Here's the drawing with two shaded views (mm, measured from the low corner). I have some questions. A direction names the side the tool comes from. Coordinates: 2 decimals unless noted, no trailing zeros. Write each loop counter-clockwise with the first axis right and the second up, starting at its lowest first coordinate (ties: lowest second). Pieces come first, ordered by that corner, then holes.
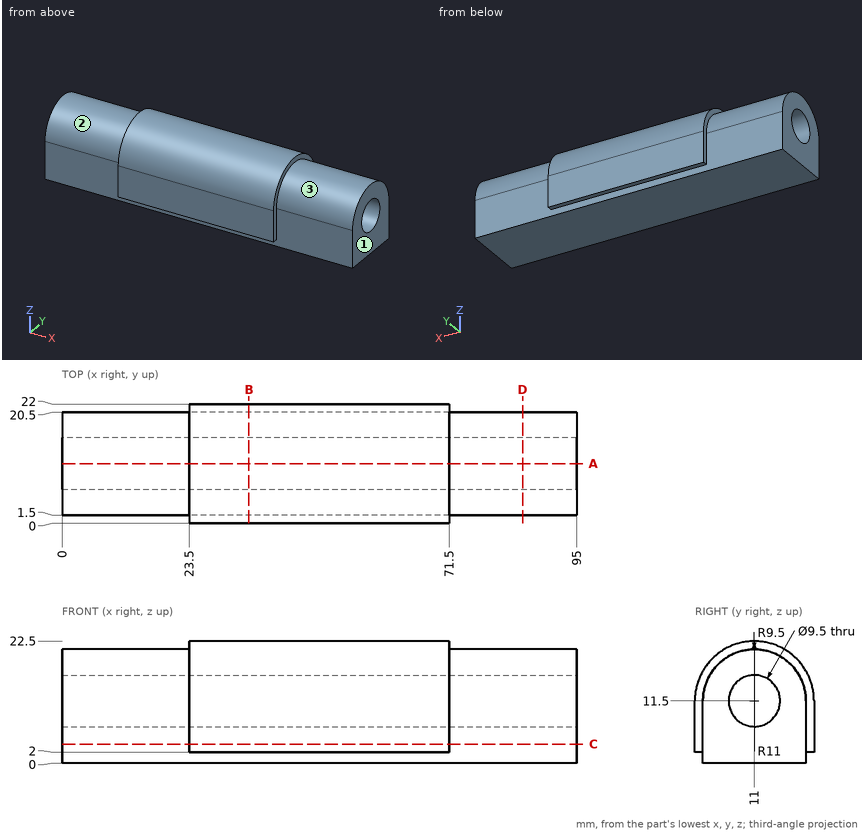
1. Which directions (+Z, -Z, +X, -X, +Y, -Y) give clear straight access to the entire face, cutting with the end or side of a thin tool? Please do the marked faces 1, 2 and 3.
2. If we section it at C-C, the plane z = 3.5: List the corners of the cut face in (x, y) for me, plus the area to 3 significant figures.
3. I'm going to push flat-ended pins straight in: P1, Ø8, axis at x = 19, y = 15, coming from the +Z side; P2, Ø8, axis at x = 18.5, z = 15, coming from the -Y side; P3, Ø0.8, axis at x = 56.5, y = 1, coming from the -Z side; P4, Ø6, axis at y = 11, z = 12.5, coming from the -X side. Where does each tip first touch, or does it pass through?
4. If we section it at B-B, the plane x = 34.5: List the corners of the cut face in (y, z) for me.
5. If we section it at A-A, the plane y = 11: List the corners of the cut face in (x, z) for me.
6. If we section it at D-D, the plane x = 85: List the corners of the cut face in (y, z) for me.
7. If I drill on L1, parallel to Z at x = 50, y = 11; L2, parallel to Z at x = 53, y = 9.5; L3, parallel to Y at x = 66, z = 11, over which ranges is the centre line in solid material (lowest first)?
Answers:
1. face 1: +Z, -Z, +X, +Y, -Y
1. face 2: +Z, -X
1. face 3: +Z, +X
2. outline: (0, 1.5) - (23.5, 1.5) - (23.5, 0) - (71.5, 0) - (71.5, 1.5) - (95, 1.5) - (95, 20.5) - (71.5, 20.5) - (71.5, 22) - (23.5, 22) - (23.5, 20.5) - (0, 20.5) - close
2. area: 1,950 mm2
3. P1: stops at z = 21
3. P2: stops at y = 1.5
3. P3: stops at z = 2
3. P4: passes through
4. outline: (0, 2) - (1.5, 2) - (1.5, 0) - (20.5, 0) - (20.5, 2) - (22, 2) - (22, 11.5) arc R11 ccw to (0, 11.5) - close; hole circle Ø9.5 at (11, 11.5)
5. outline: (0, 0) - (95, 0) - (95, 6.75) - (0, 6.75) - close; (0, 16.25) - (95, 16.25) - (95, 21) - (71.5, 21) - (71.5, 22.5) - (23.5, 22.5) - (23.5, 21) - (0, 21) - close
6. outline: (1.5, 0) - (20.5, 0) - (20.5, 11.5) arc R9.5 ccw to (1.5, 11.5) - close; hole circle Ø9.5 at (11, 11.5)
7. L1: z = 0 to 6.75, 16.25 to 22.5
7. L2: z = 0 to 6.99, 16.01 to 22.4
7. L3: y = 0 to 6.28, 15.72 to 22
